Design review of the part built by this model. Coordinates are the model's own, in mm. Face numbers are marked on the shaded views. Coordinates: 2 decimals unless noted, no trailing zeros. Loops run counter-clockwise (first coordinate to the right, second up) from the corner with the lowest first, then second, coordinate; pieces in that order, holes last. Notation, with made-up numbers: (45, 37) -> (64, 37) arc R26 ccw to (64, 61) -> close; hole circle Ø10 at (-2, 35.5). An arc over 180 degrees is marked (long way). Use one line per item in the form item = value. Start each with the question number.
1. Consider section B-B (z = 0). State the section outline as (x, y) points, then the cut area to 3 significant figures.
2. The part is to be moulded in two halves that separate along Z. For the marked faces 1, 2 and 3, say which applies: released by +Z, released by -Z, zero draft, split by the parting line, or undercut.
3. Consider section D-D (y = -10). State the section outline as (x, z) points, then the cut area to 3 significant figures.
4. Consider section C-C (x = 3). State the section outline as (y, z) points.
5. Consider section A-A (y = 0). State the section outline as (x, z) points.
6. Wall thickness on line 1 (Z direction, x = 6, y = 0.5); line 2 (Z direction, x = 2.25, y = -2); line 3 (Z direction, x = 0.5, y = 10): over which ranges is each line inside the solid? List them lowest first. Write a range as from..to.
7. For pin 1 (1 mm diameter, centred on x = 3.5, y = 3.5, fed in from -Z); pin 2 (3.5 mm diameter, centred on y = 0, z = -32, fed in from +X); pin 3 (2 mm diameter, centred on x = 1.5, y = -7, fed in from -Z); pin 4 (4 mm diameter, centred on x = 3, z = -30.5, fed in from +Y), all flat-tipped, find the tip position at first contact; note any pin that passes through.
Autodesk Inventor part; units mm, degrees
ref_plane "YZ Plane" through (0, 0, 0) normal (1, 0, 0) x (0, 1, 0)
ref_plane "XZ Plane" through (0, 0, 0) normal (0, 1, 0) x (-1, 0, 0)
ref_plane "XY Plane" through (0, 0, 0) normal (0, 0, 1) x (1, 0, 0)
sketch "Sketch4" plane through (0, 0, 0) normal (1, 0, 0) x (0, 1, 0)
  circle A0 centre (0, 0) radius 12.5
  arc A1 (-7.4162, -35) -> (7.4162, -35) centre (0, -32) ccw
  arc A2 (7.4162, 35) -> (-7.4162, 35) centre (0, 32) ccw
  line L0 (7.4162, 35) -> (18.5405, 7.5)
  line L1 (-7.4162, 35) -> (-18.5405, 7.5)
  line L2 (-18.5405, -7.5) -> (-7.4162, -35)
  line L3 (7.4162, -35) -> (18.5405, -7.5)
  arc A3 (-18.5405, 7.5) -> (-18.5405, -7.5) centre (0, 0) ccw
  arc A4 (18.5405, -7.5) -> (18.5405, 7.5) centre (0, 0) ccw
  circle A5 centre (0, 32) radius 2.25
  circle A6 centre (0, -32) radius 2.25
  line L4 (0, 32) -> (0, 0) construction
  line L5 (0, 0) -> (0, -32) construction
  dimension "d32" = 4.5
  dimension "d33" = 4.5
  dimension "d34" = 25
  dimension "d35" = 8
  dimension "d36" = 64
  dimension "d37" = 20
extrude "Extrusion2" add sketch "Sketch4" along normal blind 8
properties part number "M14 - Upper Bearing Support" material "Polycarbonate, Clear"
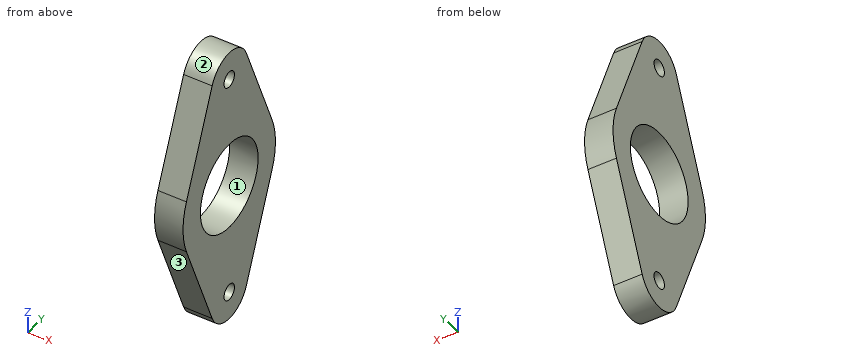
Geometry check:
q1.outline = (0, -20) -> (8, -20) -> (8, -12.5) -> (0, -12.5) -> close; (0, 12.5) -> (8, 12.5) -> (8, 20) -> (0, 20) -> close
q1.area = 120 mm²
q2.face_1 = undercut
q2.face_2 = released by +Z
q2.face_3 = released by -Z
q3.outline = (0, -28.61) -> (8, -28.61) -> (8, -7.5) -> (0, -7.5) -> close; (0, 7.5) -> (8, 7.5) -> (8, 28.61) -> (0, 28.61) -> close
q3.area = 338 mm²
q4.outline = (-18.54, -7.5) -> (-7.42, -35) arc R8 ccw to (7.42, -35) -> (18.54, -7.5) arc R20 ccw to (18.54, 7.5) -> (7.42, 35) arc R8 ccw to (-7.42, 35) -> (-18.54, 7.5) arc R20 ccw to start; hole circle Ø25 at (0, 0); hole circle Ø4.5 at (0, -32); hole circle Ø4.5 at (0, 32)
q5.outline = (0, -40) -> (8, -40) -> (8, -34.25) -> (0, -34.25) -> close; (0, -29.75) -> (8, -29.75) -> (8, -12.5) -> (0, -12.5) -> close; (0, 12.5) -> (8, 12.5) -> (8, 29.75) -> (0, 29.75) -> close; (0, 34.25) -> (8, 34.25) -> (8, 40) -> (0, 40) -> close
q6.line_1 = -39.98..-34.19, -29.81..-12.49, 12.49..29.81, 34.19..39.98
q6.line_2 = -39.75..-33.03, -30.97..-12.34, 12.34..30.97, 33.03..39.75
q6.line_3 = -28.61..-7.5, 7.5..28.61
q7.pin_1 = -39.42
q7.pin_2 = through
q7.pin_3 = -37.29
q7.pin_4 = 10.05
